from build123d import *

# Parameters (mm, degrees)
SKETCH1_W           = 22.6
SKETCH1_H           = 12.1
BOSS_EXTRUDE1_DEPTH = 22.3
SKETCH2_W           = 12.1
SKETCH2_H           = 2.5
BOSS_EXTRUDE2_DEPTH = 5
BOSS_EXTRUDE3_DEPTH = 5.5
SKETCH4_R           = 2.25
BOSS_EXTRUDE4_DEPTH = 4
CUT_EXTRUDE1_REACH  = 29.033
FILLET1_R           = 0.5


with BuildPart() as part:
    # Sketch1 → Boss-Extrude1 (new body)
    with BuildSketch(Plane(origin=(0, 0, 0), x_dir=(1, 0, 0), z_dir=(0, 1, 0))):
        Rectangle(SKETCH1_W, SKETCH1_H)
    extrude(amount=BOSS_EXTRUDE1_DEPTH)

    # Sketch2 → Boss-Extrude2 (add)
    with BuildSketch(Plane(origin=(11.3, 0, 0), x_dir=(0, 0, -1), z_dir=(1, 0, 0))):
        with Locations((0, 19.45)):
            Rectangle(SKETCH2_W, SKETCH2_H)
    boss_extrude2 = extrude(amount=BOSS_EXTRUDE2_DEPTH)

    # Mirror1: Boss-Extrude2 across plane
    add(boss_extrude2.mirror(Plane(origin=(0, 0, 0), x_dir=(0, 0, 1), z_dir=(1, 0, 0))))

    # Sketch3 → Boss-Extrude3 (add)
    with BuildSketch(Plane(origin=(0, 22.3, 0), x_dir=(1, 0, 0), z_dir=(0, 1, 0))):
        with BuildLine():
            ThreePointArc((-0.8, 3.25), (-4.05, 0), (-0.8, -3.25))
            Line((-0.8, -3.25), (0.147059671, -3.25))
            ThreePointArc((0.147059671, -3.25), (11.3, 0), (0.147059671, 3.25))
            Line((0.147059671, 3.25), (-0.8, 3.25))
        make_face()
    extrude(amount=BOSS_EXTRUDE3_DEPTH)

    # Sketch4 → Boss-Extrude4 (add)
    with BuildSketch(Plane(origin=(0, 27.8, 0), x_dir=(1, 0, 0), z_dir=(0, 1, 0))):
        with Locations(Location((5.25, 0, 0), (0, 0, 270))):
            Circle(SKETCH4_R)
    extrude(amount=BOSS_EXTRUDE4_DEPTH)

    # Sketch6 → Cut-Extrude1 (cut, up to next)
    with BuildSketch(Plane(origin=(0, 20.7, 0), x_dir=(1, 0, 0), z_dir=(0, 1, 0)), mode=Mode.PRIVATE) as cut_extrude1_sk1:
        with BuildLine():
            Line((16.3, -0.5), (16.3, 0))
            Line((16.3, 0), (15.05, 0))
            ThreePointArc((15.05, 0), (15.023632891, -0.255387055), (14.945643924, -0.5))
            Line((14.945643924, -0.5), (16.3, -0.5))
        make_face()
    cut_extrude1_tool1 = extrude(cut_extrude1_sk1.sketch, amount=-CUT_EXTRUDE1_REACH, mode=Mode.PRIVATE) & part.part
    # Sketch6 → Cut-Extrude1 (cut, up to next)
    with BuildSketch(Plane(origin=(0, 20.7, 0), x_dir=(1, 0, 0), z_dir=(0, 1, 0)), mode=Mode.PRIVATE) as cut_extrude1_sk2:
        with BuildLine():
            Line((15.05, 0), (16.3, 0))
            Line((16.3, 0), (16.3, 0.5))
            Line((16.3, 0.5), (14.945643924, 0.5))
            ThreePointArc((14.945643924, 0.5), (15.023632891, 0.255387055), (15.05, 0))
        make_face()
    cut_extrude1_tool2 = extrude(cut_extrude1_sk2.sketch, amount=-CUT_EXTRUDE1_REACH, mode=Mode.PRIVATE) & part.part
    # Sketch6 → Cut-Extrude1 (cut, up to next)
    with BuildSketch(Plane(origin=(0, 20.7, 0), x_dir=(1, 0, 0), z_dir=(0, 1, 0)), mode=Mode.PRIVATE) as cut_extrude1_sk3:
        with BuildLine():
            ThreePointArc((14.945643924, -0.5), (15.023632891, -0.255387055), (15.05, 0))
            Line((15.05, 0), (12.55, 0))
            ThreePointArc((12.55, 0), (13.544612945, -1.223632891), (14.945643924, -0.5))
        make_face()
    cut_extrude1_tool3 = extrude(cut_extrude1_sk3.sketch, amount=-CUT_EXTRUDE1_REACH, mode=Mode.PRIVATE) & part.part
    # Sketch6 → Cut-Extrude1 (cut, up to next)
    with BuildSketch(Plane(origin=(0, 20.7, 0), x_dir=(1, 0, 0), z_dir=(0, 1, 0)), mode=Mode.PRIVATE) as cut_extrude1_sk4:
        with BuildLine():
            Line((12.55, 0), (15.05, 0))
            ThreePointArc((15.05, 0), (15.023632891, 0.255387055), (14.945643924, 0.5))
            ThreePointArc((14.945643924, 0.5), (13.544612945, 1.223632891), (12.55, 0))
        make_face()
    cut_extrude1_tool4 = extrude(cut_extrude1_sk4.sketch, amount=-CUT_EXTRUDE1_REACH, mode=Mode.PRIVATE) & part.part
    # Sketch6 → Cut-Extrude1 (cut, up to next)
    with BuildSketch(Plane(origin=(0, 20.7, 0), x_dir=(1, 0, 0), z_dir=(0, 1, 0)), mode=Mode.PRIVATE) as cut_extrude1_sk5:
        with BuildLine():
            ThreePointArc((14.945643924, -0.5), (15.023632891, -0.255387055), (15.05, 0))
            Line((15.05, 0), (12.55, 0))
            ThreePointArc((12.55, 0), (13.544612945, -1.223632891), (14.945643924, -0.5))
        make_face()
    cut_extrude1_tool5 = extrude(cut_extrude1_sk5.sketch, amount=-CUT_EXTRUDE1_REACH, mode=Mode.PRIVATE) & part.part
    # Sketch6 → Cut-Extrude1 (cut, up to next)
    with BuildSketch(Plane(origin=(0, 20.7, 0), x_dir=(1, 0, 0), z_dir=(0, 1, 0)), mode=Mode.PRIVATE) as cut_extrude1_sk6:
        with BuildLine():
            Line((12.55, 0), (15.05, 0))
            ThreePointArc((15.05, 0), (15.023632891, 0.255387055), (14.945643924, 0.5))
            ThreePointArc((14.945643924, 0.5), (13.544612945, 1.223632891), (12.55, 0))
        make_face()
    cut_extrude1_tool6 = extrude(cut_extrude1_sk6.sketch, amount=-CUT_EXTRUDE1_REACH, mode=Mode.PRIVATE) & part.part
    cut_extrude1_1 = cut_extrude1_tool1.solids().sort_by_distance((15.657536, 20.7, 0.253356))[0]
    add(cut_extrude1_1, mode=Mode.SUBTRACT)
    cut_extrude1_2 = cut_extrude1_tool2.solids().sort_by_distance((15.657536, 20.7, -0.253356))[0]
    add(cut_extrude1_2, mode=Mode.SUBTRACT)
    cut_extrude1_3 = cut_extrude1_tool3.solids().sort_by_distance((13.8, 20.7, 0.530516))[0]
    add(cut_extrude1_3, mode=Mode.SUBTRACT)
    cut_extrude1_4 = cut_extrude1_tool4.solids().sort_by_distance((13.8, 20.7, -0.530516))[0]
    add(cut_extrude1_4, mode=Mode.SUBTRACT)
    cut_extrude1_5 = cut_extrude1_tool5.solids().sort_by_distance((13.8, 20.7, 0.530516))[0]
    add(cut_extrude1_5, mode=Mode.SUBTRACT)
    cut_extrude1_6 = cut_extrude1_tool6.solids().sort_by_distance((13.8, 20.7, -0.530516))[0]
    add(cut_extrude1_6, mode=Mode.SUBTRACT)
    cut_extrude1 = cut_extrude1_1 + cut_extrude1_2 + cut_extrude1_3 + cut_extrude1_4 + cut_extrude1_5 + cut_extrude1_6  # Cut-Extrude1 as one shape, for the pattern or mirror that repeats it

    # Mirror2: Cut-Extrude1 across plane
    add(cut_extrude1.mirror(Plane(origin=(0, 0, 0), x_dir=(0, 0, 1), z_dir=(1, 0, 0))), mode=Mode.SUBTRACT)

    # Fillet1
    fillet1_edges = [part.edges().sort_by_distance(p)[0] for p in [
        (16.3, 19.45, -6.05),
        (16.3, 19.45, 6.05),
        (-16.3, 19.45, -6.05),
        (-16.3, 19.45, 6.05),
    ]]
    fillet(fillet1_edges, radius=FILLET1_R)


solid = part.part
Here's how the part is built. I have some questions about the finished solid (model axes, mm). A direction names the side the tool comes from. Coordinates: 2 decimals unless noted, no trailing zeros. Write each loop counter-clockwise with the first axis right and the second up, starting at its lowest first coordinate (ties: lowest second). Pieces come first, ordered by that corner, then holes.
Item 1: I want a section at A-A on x = 13.5. Write out the boundary of the cut face in (y, z).
Item 2: If I drill on line 1 (Y direction, x = -8.5, z = 4.25); line 2 (X direction, y = 14.5, z = 3.75); line 3 (Y direction, x = 12, z = 4), over which ranges is the centre line in solid material (lowest first)?
Item 3: I want a section at B-B on z = 3.75. Write out the boundary of the cut face in (x, y), and give its area (3 significant figures).
Item 4: Will these pins go through, and if not, where does the flat tip stop? pin 1 (5.5 mm diameter, centred on x = -15, z = -1, fed in from +Y); pin 2 (4 mm diameter, centred on x = -7.5, z = 0.5, fed in from +Y); pin 3 (0.5 mm diameter, centred on x = 0, y = 26, fed in from +Z).
Item 5: I want a section at D-D on x = -12. Write out the boundary of the cut face in (y, z), and give its area (4 significant figures).
Item 6: On a 3-axis mill with a long thin cutter (end or side, diameter ignored), from which of +Z, -Z, +X, -X, +Y, -Y can I reach the whole of each face in a straight line? I mean faces 1 (the flat face through (16, 19, -0.5)), 2 (the flat face through (-5, 22.3, 0)), 3 (the cylindrical face through (11.296, 25.012, 0.218)), 4 (the flat face through (-0.3, 25, -3.25)). Say none if no direction works.
Item 7: I want a section at C-C on y = 11. Write out the boundary of the cut face in (x, z), and give its area (3 significant figures).
Findings below:
1. outline: (18.2, -6.05) - (20.7, -6.05) - (20.7, -1.21) - (18.2, -1.21) - close; (18.2, 1.21) - (20.7, 1.21) - (20.7, 6.05) - (18.2, 6.05) - close
2. line 1: y = 0 to 22.3
2. line 2: x = -11.3 to 11.3
2. line 3: y = 18.2 to 20.7
3. outline: (-16.3, 18.2) - (-11.3, 18.2) - (-11.3, 0) - (11.3, 0) - (11.3, 18.2) - (16.3, 18.2) - (16.3, 20.7) - (11.3, 20.7) - (11.3, 22.3) - (10, 22.3) - (10, 27.8) - (0.5, 27.8) - (0.5, 22.3) - (-11.3, 22.3) - (-11.3, 20.7) - (-16.3, 20.7) - close
3. area: 581 mm2
4. pin 1: stops at y = 20.7
4. pin 2: stops at y = 22.3
4. pin 3: stops at z = 3.41
5. outline: (18.2, -6.05) - (20.7, -6.05) - (20.7, 6.05) - (18.2, 6.05) - close
5. area: 30.25 mm2
6. face 1: +X, +Y, -Y
6. face 2: -X, +Y
6. face 3: +Y
6. face 4: -Z, -X, +Y
7. outline: (-11.3, -6.05) - (11.3, -6.05) - (11.3, 6.05) - (-11.3, 6.05) - close
7. area: 273 mm2
